The listing builds one solid part. Answer for the finished solid, in the listing's coordinates (mm). Face numbers are marked on the shaded views. A direction names the side the tool comes from. Give positions to 0.01 mm unless a question says otherwise; leave off trailing zeros. Write each loop counter-clockwise with the first axis right and the second up, starting at its lowest first coordinate (ties: lowest second). Pieces come first, ordered by that corner, then holes. Notation, with made-up numbers: (-1.5, 76.25) - (34.5, 76.25) arc R24 ccw to (34.5, 112.25) - close; hole circle Ø3 at (48.25, 82.25). An arc over 180 degrees is marked (long way). Return JSON: item names as keys, results as strings.
from build123d import *

# Parameters (mm, degrees)
SKETCH1_R           = 9.25
BOSS_EXTRUDE1_DEPTH = 40
SKETCH2_R           = 8
BOSS_EXTRUDE2_DEPTH = 90
BOSS_EXTRUDE3_START = 30
SKETCH3_R           = 8
BOSS_EXTRUDE3_DEPTH = 30
SKETCH4_R           = 6.75
BOSS_EXTRUDE4_DEPTH = 35
SKETCH5_R           = 4.5
BOSS_EXTRUDE5_DEPTH = 30
CUT_EXTRUDE1_START  = -5
SKETCH6_W           = 3
SKETCH6_H           = 6
CUT_EXTRUDE1_DEPTH  = 20
CUT_EXTRUDE2_START  = -65
SKETCH7_W           = 5
SKETCH7_H           = 6
CUT_EXTRUDE2_DEPTH  = 20


with BuildPart() as part:
    # Sketch1 → Boss-Extrude1 (new body)
    with BuildSketch(Plane.XY):
        Circle(SKETCH1_R)
    extrude(amount=BOSS_EXTRUDE1_DEPTH)

    # Sketch2 → Boss-Extrude2 (add)
    with BuildSketch(Plane.XY.offset(40)):
        with Locations(Location((0, 0, 0), (0, 0, 180))):
            Circle(SKETCH2_R)
    extrude(amount=BOSS_EXTRUDE2_DEPTH)

    # Sketch3 → Boss-Extrude3 (add)
    with BuildSketch(Plane(origin=(0, 0, 0), x_dir=(-1, 0, 0), z_dir=(0, 0, -1)).offset(BOSS_EXTRUDE3_START)):
        Circle(SKETCH3_R)
    extrude(amount=-BOSS_EXTRUDE3_DEPTH)

    # Sketch4 → Boss-Extrude4 (add)
    with BuildSketch(Plane.XY.offset(130)):
        Circle(SKETCH4_R)
    extrude(amount=BOSS_EXTRUDE4_DEPTH)

    # Sketch5 → Boss-Extrude5 (add)
    with BuildSketch(Plane.XY.offset(165)):
        Circle(SKETCH5_R)
    extrude(amount=BOSS_EXTRUDE5_DEPTH)

    # Sketch6 → Cut-Extrude1 (cut)
    with BuildSketch(Plane.XY.offset(195).offset(CUT_EXTRUDE1_START)):
        with Locations((0, 4.5)):
            Rectangle(SKETCH6_W, SKETCH6_H)
    extrude(amount=-CUT_EXTRUDE1_DEPTH, mode=Mode.SUBTRACT)

    # Sketch7 → Cut-Extrude2 (cut)
    with BuildSketch(Plane.XY.offset(130).offset(CUT_EXTRUDE2_START)):
        with Locations((0, 8)):
            Rectangle(SKETCH7_W, SKETCH7_H)
    extrude(amount=-CUT_EXTRUDE2_DEPTH, mode=Mode.SUBTRACT)


solid = part.part
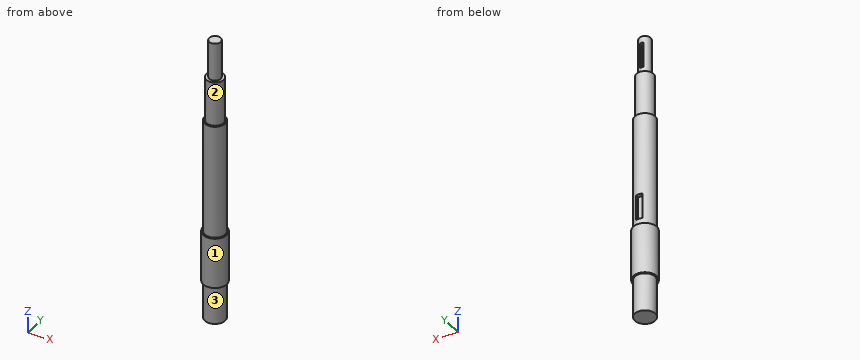
Item 1: Flat-ended cylindrical pins translate along their axes: P1, Ø2.5, axis at x = 0, z = 179.5, coming from the +Y side; P2, Ø6, axis at y = 4.5, z = 75, coming from the -X side; P3, Ø4, axis at x = 0.5, z = 19, coming from the -Y side; P4, Ø3, axis at y = 2.5, z = 177.5, coming from the +X side. Find the tip coordinate at first contact, or state that the pin passes through.
Answer below:
{"P1": "stops at y = 1.5", "P2": "stops at x = -7.86", "P3": "stops at y = -9.25", "P4": "stops at x = 4.39"}
Item 2: Consider L1, parallel to Z at x = -0.25, y = 6.5; L2, parallel to Z at x = 3.25, y = 3.25; L3, parallel to Z at x = -7.75, y = -0.5. Determine where each line is inside the solid, lowest interval first.
Answer below:
{"L1": "z = -30 to 45, 65 to 165", "L2": "z = -30 to 165", "L3": "z = -30 to 130"}
Item 3: For the marked faces 1, 2 and 3, determine the directions among +Z, -Z, +X, -X, +Y, -Y from which every point of the face is accessible in a straight line to the end or side of a thin tool.
Answer below:
{"face 1": "+Z, -Z", "face 2": "+Z", "face 3": "-Z"}
Item 4: A cutting plane is placed at A-A on z = 78.5. Determine the outline of the cut face in (x, y), then the cut area to 3 significant figures.
Answer below:
{"outline": "circle Ø16 at (0, 0)", "area": "201 mm²"}
